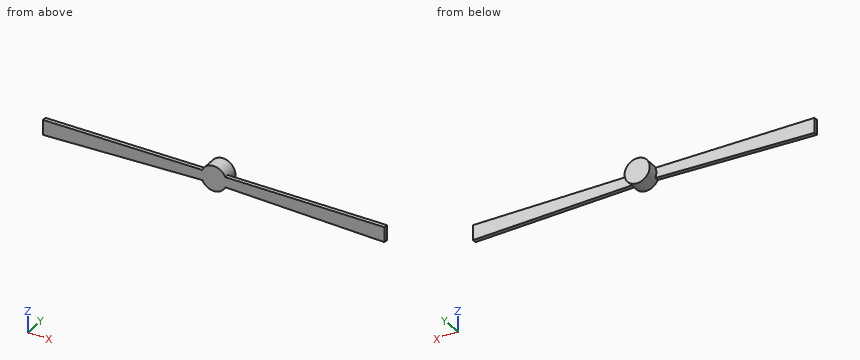
```python
from build123d import *

# Parameters (mm, degrees)
SKETCH1_R           = 25
BOSS_EXTRUDE1_DEPTH = 30
BOSS_EXTRUDE2_DEPTH = 8


with BuildPart() as part:
    # Sketch1 → Boss-Extrude1 (new body)
    with BuildSketch(Plane(origin=(0, 0, 0), x_dir=(1, 0, 0), z_dir=(0, 1, 0))):
        with Locations(Location((0, 0, 0), (0, 0, 270))):
            Circle(SKETCH1_R)
    extrude(amount=BOSS_EXTRUDE1_DEPTH)

    # Sketch2 → Boss-Extrude2 (add)
    with BuildSketch(Plane(origin=(0, 0, 0), x_dir=(1, 0, 0), z_dir=(0, 1, 0))):
        Polygon((15, 10), (340, 20), (340, -10), (15, -10), align=None)
        Polygon((-15, 10), (-340, 20), (-340, -10), (-15, -10), align=None)
    extrude(amount=BOSS_EXTRUDE2_DEPTH)


solid = part.part
```
The listing builds one solid part. Answer for the finished solid, in the listing's coordinates (mm). Coordinates: 2 decimals unless noted, no trailing zeros. Write each loop counter-clockwise with the first axis right and the second up, starting at its lowest first coordinate (ties: lowest second). Pieces come first, ordered by that corner, then holes. Notation, with made-up numbers: (84, -10) - (125, -10) arc R23 ccw to (125, 18) - close; hole circle Ø2 at (8.5, 73.25). An arc over 180 degrees is marked (long way). Return JSON: item names as keys, results as strings. Group by question number.
1. A cutting plane is placed at D-D, the plane x = 162.5. Determine the outline of the cut face in (y, z), plus the area to 3 significant figures.
2. A cutting plane is placed at A-A, the plane z = 0. Determine the outline of the cut face in (x, y), plus the area to 3 significant figures.
3. Given pin 1 (5 mm diameter, centred on x = -236, y = 8.5, fed in from +Z); pin 2 (8 mm diameter, centred on y = 26.5, z = -14.5, fed in from -X); pin 3 (1 mm diameter, centred on x = 184.5, y = 5.5, fed in from -Z), each flat-ended and moving along its own axis, determine where each tip first touches the part or whether it passes through.
4. A cutting plane is placed at C-C, the plane y = 25.25. Determine the outline of the cut face in (x, z).
5. A cutting plane is placed at B-B, the plane x = -235.5. Determine the outline of the cut face in (y, z).
6. Straight lines are drawn through the part: L1, parallel to Y at x = 236, z = -2; L2, parallel to X at y = 15.75, z = 0; L3, parallel to X at y = 21, z = 19. For each, find the intervals that lie inside material, in ascending order.
Ans:
{
 "1": {"outline": "(0, -14.54) - (8, -14.54) - (8, 10) - (0, 10) - close", "area": "196 mm²"},
 "2": {"outline": "(-340, 0) - (340, 0) - (340, 8) - (25, 8) - (25, 30) - (-25, 30) - (-25, 8) - (-340, 8) - close", "area": "6,540 mm²"},
 "3": {"pin 1": "z = 10", "pin 2": "x = -22.69", "pin 3": "z = -15.23"},
 "4": {"outline": "circle Ø50 at (0, 0)"},
 "5": {"outline": "(0, -16.78) - (8, -16.78) - (8, 10) - (0, 10) - close"},
 "6": {"L1": "0 to 8", "L2": "-25 to 25", "L3": "-16.25 to 16.25"}
}
